The listing builds one solid part. Answer for the finished solid, in the listing's coordinates (mm). A direction names the side the tool comes from. Coordinates: 2 decimals unless noted, no trailing zeros. Order: outer loops, then holes, each group sorted by start corner. A loop starts at its lowest first (then second) coordinate and runs counter-clockwise, first axis right, second up. Notation, with made-up numbers: (1, 19) -> (27, 19) arc R9 ccw to (27, 24) -> close; hole circle Ø4 at (20.5, 5.5). An arc over 180 degrees is marked (long way). Put each result on its own line as item: value. Start each with the question number.
```python
from build123d import *

# Parameters (mm, degrees)
SKETCH1_W                = 69
SKETCH1_H                = 13
BOSS_EXTRUDE1_DEPTH      = 1.6
SKETCH2_W                = 69
SKETCH2_H                = 2
BOSS_EXTRUDE2_DEPTH      = 7.3
FILLET1_R                = 1
M2_START                 = -6.5
M2_CLEARANCE_SLOT1_DEPTH = 2


# Read off the part's stored shape, not the designer's step: M2 Clearance Slot1
with BuildPart() as part:
    # Sketch1 → Boss-Extrude1 (new body)
    with BuildSketch(Plane(origin=(0, 0, 0), x_dir=(1, 0, 0), z_dir=(0, 1, 0))):
        Rectangle(SKETCH1_W, SKETCH1_H)
    extrude(amount=BOSS_EXTRUDE1_DEPTH)

    # Sketch2 → Boss-Extrude2 (add)
    with BuildSketch(Plane(origin=(0, 1.6, 0), x_dir=(1, 0, 0), z_dir=(0, 1, 0))):
        with Locations((0, 5.5)):
            Rectangle(SKETCH2_W, SKETCH2_H)
    extrude(amount=BOSS_EXTRUDE2_DEPTH)

    # Fillet1
    fillet1_edges = [part.edges().sort_by_distance(p)[0] for p in [
        (0, 1.6, -4.5),
    ]]
    fillet(fillet1_edges, radius=FILLET1_R)

    # M2 Clearance Slot1 outline → M2 Clearance Slot1 (cut)
    with BuildSketch(Plane.XY.offset(M2_START)):
        with BuildLine():
            Line((23.2, 3.8), (23.2, 5.4))
            ThreePointArc((23.2, 5.4), (22, 6.6), (20.8, 5.4))
            Line((20.8, 5.4), (20.8, 3.8))
            ThreePointArc((20.8, 3.8), (22, 2.6), (23.2, 3.8))
        make_face()
        with BuildLine():
            Line((1.2, 3.8), (1.2, 5.4))
            ThreePointArc((1.2, 5.4), (0, 6.6), (-1.2, 5.4))
            Line((-1.2, 5.4), (-1.2, 3.8))
            ThreePointArc((-1.2, 3.8), (0, 2.6), (1.2, 3.8))
        make_face()
        with BuildLine():
            Line((-20.8, 3.8), (-20.8, 5.4))
            ThreePointArc((-20.8, 5.4), (-22, 6.6), (-23.2, 5.4))
            Line((-23.2, 5.4), (-23.2, 3.8))
            ThreePointArc((-23.2, 3.8), (-22, 2.6), (-20.8, 3.8))
        make_face()
    extrude(amount=M2_CLEARANCE_SLOT1_DEPTH, mode=Mode.SUBTRACT)


solid = part.part
```
(1) Each of these flat-tipped pins is pushed along its axis until it touches: P1, Ø5, axis at x = 7.5, z = 0.5, coming from the +Y side; P2, Ø1, axis at y = 3, z = -1, coming from the +X side. Where does it stop, or does it pass through?
(2) The part is cut by section A-A on y = 4.75. Determine the outline of the cut face in (x, z), plus the area to 3 significant figures.
(3) The part is cut by section B-B on x = -18.5. Determine the outline of the cut face in (y, z).
(4) For a pull along X with two mould halves and no side action, classify faces 4 (the flat face through (34.5, 1, -2)), 5 (the cylindrical face through (22, 6.6, -5.5)), 6 (the flat face through (0, 2, -6.5)), 7 (the flat face through (-20.8, 5, -6)) as released by +X, released by -X, zero draft, split by the parting line, or undercut.
(5) The part is cut by section D-D on y = 8.25. Determine the outline of the cut face in (x, z), plus the area to 3 significant figures.
(6) A tool of negligible diameter and unlimited length cuts with its end or side. For faces 1 (the flat face through (0, 7, -4.5)), 2 (the cylindrical face through (-22, 2.6, -5.5)), 3 (the flat face through (0, 1, 6.5)), from which of +Z, -Z, +X, -X, +Y, -Y can it reach the whole face along a straight path? Write none if from no direction.
(7) The part is cut by section C-C on z = -1.75. Determine the outline of the cut face in (x, y), plus the area to 3 significant figures.
(8) Find the intervals of material crossed by L1, parallel to Y at x = -9, z = 2.5; L2, parallel to Z at x = 7.5, y = 8; L3, parallel to Z at x = 16.5, y = 2.25, in increasing order.
Worked out:
1. P1: y = 1.6
1. P2: through
2. outline: (-34.5, -6.5) -> (-23.2, -6.5) -> (-23.2, -4.5) -> (-34.5, -4.5) -> close; (-20.8, -6.5) -> (-1.2, -6.5) -> (-1.2, -4.5) -> (-20.8, -4.5) -> close; (1.2, -6.5) -> (20.8, -6.5) -> (20.8, -4.5) -> (1.2, -4.5) -> close; (23.2, -6.5) -> (34.5, -6.5) -> (34.5, -4.5) -> (23.2, -4.5) -> close
2. area: 124 mm2
3. outline: (0, -6.5) -> (8.9, -6.5) -> (8.9, -4.5) -> (2.6, -4.5) arc R1 cw to (1.6, -3.5) -> (1.6, 6.5) -> (0, 6.5) -> close
4. face 4: released by +X
4. face 5: undercut
4. face 6: zero draft
4. face 7: undercut
5. outline: (-34.5, -6.5) -> (34.5, -6.5) -> (34.5, -4.5) -> (-34.5, -4.5) -> close
5. area: 138 mm2
6. face 1: +Z, +X, -X, +Y
6. face 2: +Z, -Z
6. face 3: +Z, +X, -X, +Y, -Y
7. outline: (-34.5, 0) -> (34.5, 0) -> (34.5, 1.6) -> (-34.5, 1.6) -> close
7. area: 110 mm2
8. L1: 0 to 1.6
8. L2: -6.5 to -4.5
8. L3: -6.5 to -4.44
